Model file for the job. Use its own axes, mm. A direction names the side the tool comes from. Round coordinates to 2 decimals unless told otherwise and drop trailing zeros. Loops run counter-clockwise (first coordinate to the right, second up) from the corner with the lowest first, then second, coordinate; pieces in that order, holes last. Notation, with made-up numbers: (-21, 8) -> (12, 8) arc R18 ccw to (12, 29) -> close; hole circle Ø1 at (62, -8). An arc over 180 degrees is marked (long way). Use a Markdown table: item, result.
from build123d import *

# Parameters (mm, degrees)
SALIENTE_EXTRUIR1_DEPTH = 6
SALIENTE_EXTRUIR2_DEPTH = 3


with BuildPart() as part:
    # Croquis1 → Saliente-Extruir1 (new body)
    with BuildSketch(Plane(origin=(0, 0, 0), x_dir=(1, 0, 0), z_dir=(0, 1, 0))):
        Polygon((-3.602218893, 50), (2.544306114, 50), (66.713907176, -5), (-28.729177989, -5), (-28.729177989, 0), (6.61797667, 41.240232966), align=None)
        Polygon((-23.460968903, 0), (12.711587976, 0), (30.508284771, 20.763762429), (9.655061899, 38.637136097), align=None, mode=Mode.SUBTRACT)
        Polygon((54.733782073, 0), (33.54537, 18.160665559), (17.979797062, 0), align=None, mode=Mode.SUBTRACT)
    extrude(amount=SALIENTE_EXTRUIR1_DEPTH)

    # Croquis2 → Saliente-Extruir2 (add)
    with BuildSketch(Plane(origin=(0, 6, 0), x_dir=(1, 0, 0), z_dir=(0, 1, 0))):
        Polygon((-28.729177989, -5), (66.713907176, -5), (63.797107127, -2.5), (-28.729177989, -2.5), align=None)
    extrude(amount=SALIENTE_EXTRUIR2_DEPTH)


solid = part.part
Q1. Band-saw the part on A-A, the plane y = 5. Give the cut face in (x, z), plus the area to 3 significant figures.
Results list:
| item | result |
|---|---|
| outline | (-28.73, 0) -> (6.62, -41.24) -> (-3.6, -50) -> (2.54, -50) -> (66.71, 5) -> (-28.73, 5) -> close; hole (-23.46, 0) -> (9.66, -38.64) -> (30.51, -20.76) -> (12.71, 0) -> close; hole (17.98, 0) -> (33.55, -18.16) -> (54.73, 0) -> close |
| area | 1,080 mm² |
Q2. Band-saw the part on B-B, the plane x = 46. Give the cut face in (y, z), plus the area to 3 significant figures.
Results list:
| item | result |
|---|---|
| outline | (0, -12.75) -> (6, -12.75) -> (6, -7.49) -> (0, -7.49) -> close; (0, 0) -> (6, 0) -> (6, 2.5) -> (9, 2.5) -> (9, 5) -> (0, 5) -> close |
| area | 69.1 mm² |
Q3. Drill centre lines: L1, parallel to X at y = 1.75, z = -3; L2, parallel to X at y = 1.5, z = -7; L3, parallel to Z at x = 2.5, y = 2.75. Where is each one in solid material? Low to high. Write a range as from..to.
Results list:
| item | result |
|---|---|
| L1 | x = -26.16..-20.89, 15.28..20.55, 51.23..57.38 |
| L2 | x = -22.73..-17.46, 18.71..23.98, 46.57..52.71 |
| L3 | z = -50..-44.77, -36.44..-30.29, 0..5 |
Q4. Band-saw the part on C-C, the plane x = -2. Give the cut face in (y, z), plus the area to 3 significant figures.
Results list:
| item | result |
|---|---|
| outline | (0, -50) -> (6, -50) -> (6, -48.63) -> (0, -48.63) -> close; (0, -31.19) -> (6, -31.19) -> (6, -25.04) -> (0, -25.04) -> close; (0, 0) -> (6, 0) -> (6, 2.5) -> (9, 2.5) -> (9, 5) -> (0, 5) -> close |
| area | 82.6 mm² |
Q5. Band-saw the part on D-D, the plane z = -16. Give the cut face in (x, y).
Results list:
| item | result |
|---|---|
| outline | (-15.02, 0) -> (-9.75, 0) -> (-9.75, 6) -> (-15.02, 6) -> close; (26.43, 0) -> (31.69, 0) -> (31.69, 6) -> (26.43, 6) -> close; (36.07, 0) -> (42.21, 0) -> (42.21, 6) -> (36.07, 6) -> close |
Q6. Pull direction Z, two halves, no side cores. Call faces 4 (the face through (18, 7, 2.5)), 5 (the face through (21, 6, -8)), 6 (the face through (20.2, 3, -29.6)): released by +Z, released by -Z, zero draft, split by the parting line, or undercut.
Results list:
| item | result |
|---|---|
| face 4 | released by -Z |
| face 5 | zero draft |
| face 6 | undercut |
Q7. Tool access for faces 1 (the face through (-11.303, 2.958, -20.331)), 2 (the face through (-6.67, 2.96, -19.59)), 3 (the face through (-28.729, 3, 2)): list every direction of +Z, -Z, +X, -X, +Y, -Y with a clear straight run to the whole face (end or side of a thin tool).
Results list:
| item | result |
|---|---|
| face 1 | -X, +Y, -Y |
| face 2 | +Y, -Y |
| face 3 | +Z, -Z, -X, +Y, -Y |
Q8. Flat gauge pins, fed straight in: pin 1 (3 mm diameter, centred on x = 4.5, z = -41, fed in from +Y); pin 2 (5 mm diameter, centred on x = 44, y = 3.5, fed in from -Z). Where does each tip first touch, or does it go through?
Results list:
| item | result |
|---|---|
| pin 1 | stops at y = 6 |
| pin 2 | stops at z = -16.61 |
